For this review, take the finished solid that the model builds, in its own axes (mm). Face numbers are marked on the shaded views. A direction names the side the tool comes from. Coordinates: 2 decimals unless noted, no trailing zeros. Loops run counter-clockwise (first coordinate to the right, second up) from the corner with the lowest first, then second, coordinate; pieces in that order, holes last. Notation, with made-up numbers: M -29.75,-1.5 L -20.75,-1.5 A27 cw -20.75,34.5 Z; hole C 24,83 d2. An arc over 180 degrees is marked long. Answer as a JSON object with one key per item and string values. Group by question number.
Item 1: Add section C-C (y = 21). State the section outline as (x, z) points, then the cut area to 3 significant figures.
Item 2: Add section A-A (x = 7). State the section outline as (y, z) points.
Item 3: Insertion check: pin 1 (1 mm diameter, centred on y = 65.5, z = 2, fed in from -X); pin 2 (1 mm diameter, centred on y = 67, z = 0, fed in from +X); pin 3 (2 mm diameter, centred on y = 31.5, z = -2.5, fed in from +X). Each pin has a flat end and moves straight along its axis. Give the tip position at first contact, or say it passes through.
Item 4: Tool access review of the marked faces 1 and 2: name each direction out of +Z, -Z, +X, -X, +Y, -Y from which nothing blocks a thin tool from reaching the whole face with its end or side.
Item 5: Wall thickness on L1, parallel to X at y = 21, z = -2.4; L2, parallel to X at y = 61.5, z = 1.35; L3, parallel to Y at x = -1.5, z = -1.6: over which ranges is each line inside the solid? List them lowest first. Write a range as from..to.
Item 6: Mouldability with a two-part tool opening along X and no side actions: class the marked faces 3, 4, 5 and 6 as +X half, -X half, draft (parallel to the pull), parting line (faces both ways), or undercut.
Item 7: Add section B-B (z = 1). State the section outline as (x, y) points, then the cut area to 3 significant figures.
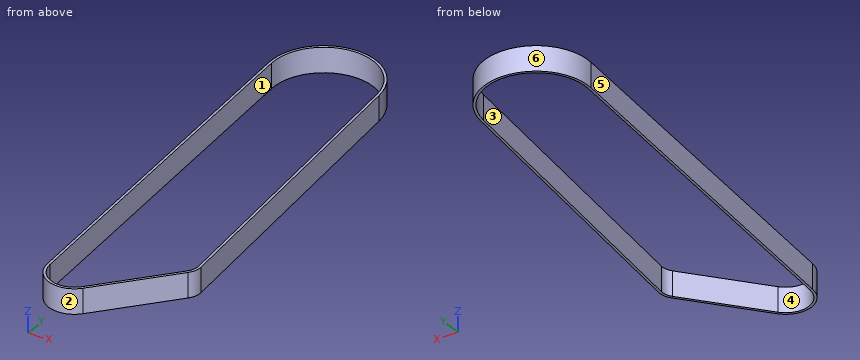
Autodesk Inventor part; units mm, degrees
ref_plane "Cross Section Plane" through (-5.9527, -0.4318, 0) normal (-0.0723, 0.9974, 0) x (0, 0, 1)
ref_plane "Work Plane2" through (0, 0, 0) normal (-1, 0, 0) x (0, 0, 1)
ref_plane "Work Plane3" through (15.5, 15.5, 0) normal (0.2665, 0.9638, 0) x (0, 0, 1)
sketch "Sketch Path" plane through (0, 0, 0) normal (0, 0, 1) x (1, 0, 0)
  arc A0 (-5.9527, -0.4318) -> (4.5858, -3.8198) centre (0, 0) ccw
  arc A1 (18.5572, 12.9535) -> (19.4599, 15.888) centre (15.5, 15.5) ccw
  arc A2 (12.2757, 89.2029) -> (-12.3022, 87.1077) centre (0, 88) ccw
  line L0 (-12.3022, 87.1077) -> (-5.9527, -0.4318)
  line L1 (4.5858, -3.8198) -> (18.5572, 12.9535)
  line L2 (19.4599, 15.888) -> (12.2757, 89.2029)
ref_plane "Cross Section Plane" through (-5.9527, -0.4318, 0) normal (-0.0723, 0.9974, 0) x (0, 0, 1)
ref_plane "Work Plane2" through (0, 0, 0) normal (-1, 0, 0) x (0, 0, 1)
ref_plane "Work Plane3" through (15.5, 15.5, 0) normal (0.2665, 0.9638, 0) x (0, 0, 1)
ref_plane "Work Plane4" through (0, 88, 0) normal (-0.286, 0.9582, 0) x (0, 0, 1)
sketch "Cross Section" plane through (-5.9527, -0.4318, 0) normal (-0.0723, 0.9974, 0) x (0, 0, 1)
  line L0 (-3, 0.3) -> (3, 0.3)
  line L1 (3, 0.3) -> (3, -0.3)
  line L2 (3, -0.3) -> (-3, -0.3)
  line L3 (-3, -0.3) -> (-3, 0.3)
  line L4 (-3, 0) -> (3, 0) construction
  point P0 (0, 0)
  point P1 (0, 0)
  dimension "d0" = 6
  dimension "d4" = 0.3
  dimension "d5" = 0.3
sweep "Belt" add profiles "Cross Section" path "Sketch Path"
equation "\"d0\" = da_B"
equation "\"d4\" = da_a"
equation "\"d5\" = da_a2"
equation "\"da_B\" = 6"
equation "\"da_pb\" = 2.5"
equation "\"da_L\" = 239.02838"
equation "\"da_a\" = 0.3"
equation "\"da_S\" = 1.5"
equation "\"da_Beta\" = 20deg"
equation "\"da_Ht\" = 0.7"
equation "\"da_H\" = 1.3"
equation "\"da_a2\" = 0.3"
properties part number "Synchronous Belt" material "Rubber"
From the geometry:
{
 "1": {"outline": "M -7.81,-3 L -7.21,-3 L -7.21,3 L -7.81,3 Z; M 18.66,-3 L 19.26,-3 L 19.26,3 L 18.66,3 Z", "area": "7.23 mm²"},
 "2": {"outline": "M -1.39,-3 L -0.45,-3 L -0.45,3 L -1.39,3 Z; M 97.79,-3 L 98.52,-3 L 98.52,3 L 97.79,3 Z"},
 "3": {"pin 1": "stops at x = -11.07", "pin 2": "stops at x = 14.8", "pin 3": "stops at x = 18.33"},
 "4": {"face 1": "+Z, -Z", "face 2": "+Z, -Z, -Y"},
 "5": {"L1": "x = -7.81..-7.21, 18.66..19.26", "L2": "x = -10.75..-10.14, 14.69..15.29", "L3": "y = -6.09..-5.47, 99.94..100.55"},
 "6": {"face 3": "undercut", "face 4": "undercut", "face 5": "-X half", "face 6": "parting line"},
 "7": {"outline": "M -12.6,87.09 L -6.25,-0.45 A6.27 ccw 4.82,-4.01 L 18.79,12.76 A4.28 ccw 19.76,15.92 L 12.57,89.23 A12.63 ccw Z; hole M -12,87.13 L -5.65,-0.41 A5.67 ccw 4.36,-3.63 L 18.33,13.15 A3.68 ccw 19.16,15.86 L 11.98,89.17 A12.03 ccw Z", "area": "143 mm²"}
}
